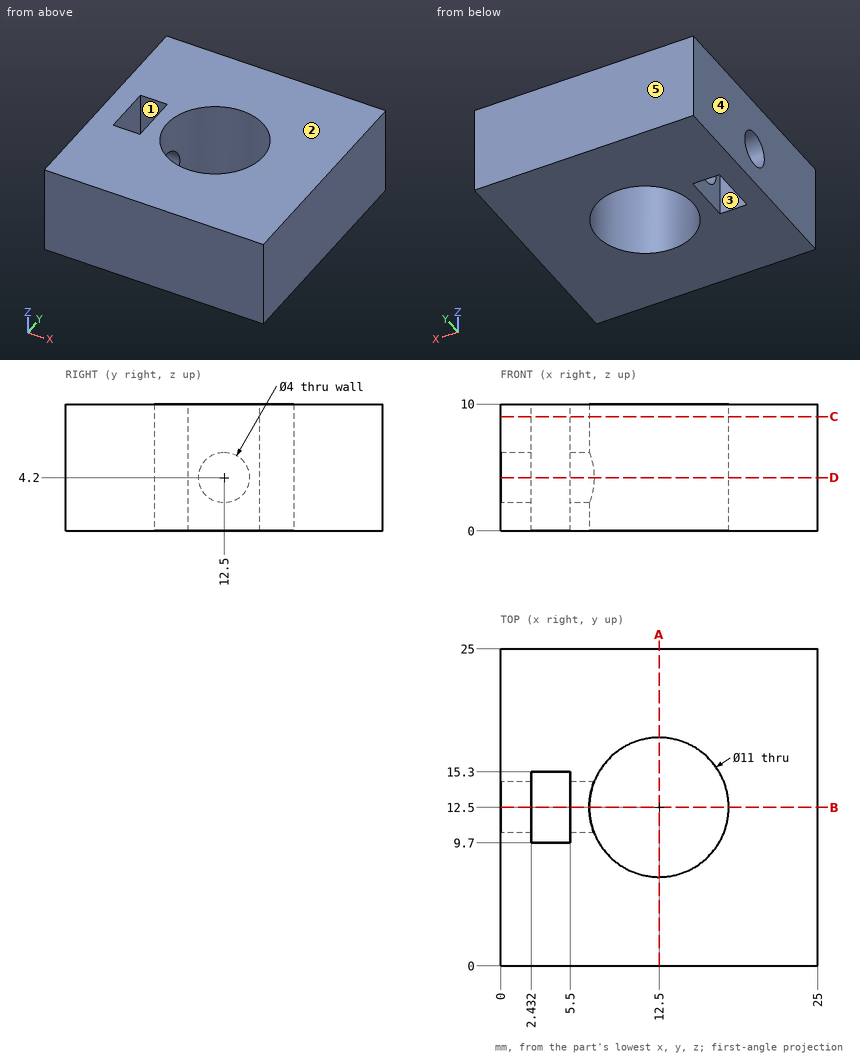
The figure shows three views and two pictorial views of one solid part (mm, origin at its lowest corner). Answer the questions. A direction names the side the tool comes from. Give positions to 0.01 mm unless a question says otherwise; leave off trailing zeros. Write each loop counter-clockwise with the first axis right and the second up, starting at its lowest first coordinate (ties: lowest second). Pieces come first, ordered by that corner, then holes.
Q1. For a pull along X with two mould halves and no side action, classify the marked faces 3, 4 and 5 as released by +X, released by -X, zero draft, split by the parting line, or undercut.
Answer:
face 3: undercut
face 4: released by -X
face 5: zero draft
Q2. The part is cut by section D-D on z = 4.2. Give the vertices of the cut face in (x, y).
Answer:
outline: (0, 0) - (25, 0) - (25, 25) - (0, 25) - (0, 14.5) - (2.43, 14.5) - (2.43, 15.3) - (5.5, 15.3) - (5.5, 14.5) - (7.38, 14.5) arc R5.5 cw (long way) to (7.38, 10.5) - (5.5, 10.5) - (5.5, 9.7) - (2.43, 9.7) - (2.43, 10.5) - (0, 10.5) - close
Q3. The part is cut by section C-C on z = 9. Give the vertices of the cut face in (x, y), and give its area (3 significant figures).
Answer:
outline: (0, 0) - (25, 0) - (25, 25) - (0, 25) - close; hole (2.43, 9.7) - (5.5, 9.7) - (5.5, 15.3) - (2.43, 15.3) - close; hole circle Ø11 at (12.5, 12.5)
area: 513 mm2
Q4. The part is cut by section B-B on y = 12.5. Give the vertices of the cut face in (x, z), and give its area (3 significant figures).
Answer:
outline: (0, 0) - (2.43, 0) - (2.43, 2.2) - (0, 2.2) - close; (0, 6.2) - (2.43, 6.2) - (2.43, 10) - (0, 10) - close; (5.5, 0) - (7, 0) - (7, 2.2) - (5.5, 2.2) - close; (5.5, 6.2) - (7, 6.2) - (7, 10) - (5.5, 10) - close; (18, 0) - (25, 0) - (25, 10) - (18, 10) - close
area: 93.6 mm2
Q5. The part is cut by section A-A on x = 12.5. Give the vertices of the cut face in (y, z).
Answer:
outline: (0, 0) - (7, 0) - (7, 10) - (0, 10) - close; (18, 0) - (25, 0) - (25, 10) - (18, 10) - close
Q6. A tool of negligible diameter and unlimited length cuts with its end or side. For the marked faces 1 and 2, from which of +Z, -Z, +X, -X, +Y, -Y can it reach the whole face along a straight path? Write none if from no direction.
Answer:
face 1: +Z, -Z
face 2: +Z, +X, -X, +Y, -Y
Q7. Straight lines are drawn through the part: L1, parallel to Y at x = 12.5, z = 5; L2, parallel to Y at x = 1.45, z = 4.2; L3, parallel to X at y = 14.25, z = 0.75. For each, find the intervals that lie inside material, in ascending order.
Answer:
L1: y = 0 to 7, 18 to 25
L2: y = 0 to 10.5, 14.5 to 25
L3: x = 0 to 2.43, 5.5 to 7.29, 17.71 to 25
